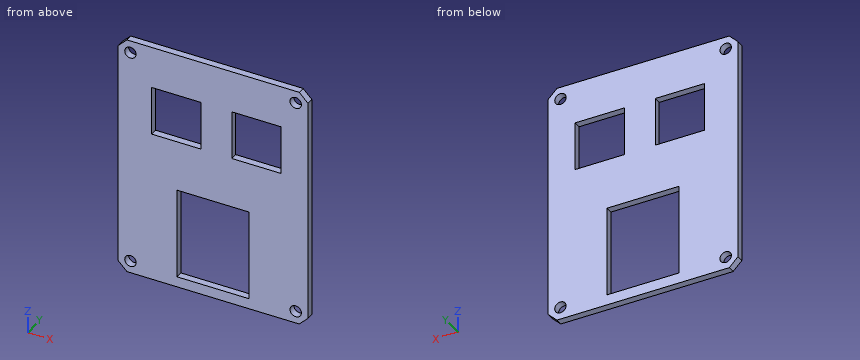
Autodesk Fusion 360 part; units mm, degrees
sketch "Sketch1" plane through (0, 0, 0) normal (0, 1, 0) x (1, 0, 0)
  line L0 (0, 0) -> (54, 0)
  line L1 (54, 0) -> (54, 69.5)
  line L2 (54, 69.5) -> (0, 69.5)
  line L3 (0, 69.5) -> (0, 0)
  dimension "d1" = 54
  dimension "d2" = 69.5
extrude "Extrude1" add sketch "Sketch1" along normal blind 2
chamfer "Chamfer1" distance 2.5 angle 45 4 edges at (54, 1, 0) (0, 1, 0) (54, 1, -69.5) (0, 1, -69.5)
sketch "Sketch2" plane through (0, 2, 0) normal (0, 1, 0) x (-1, 0, 0)
  line L0 (-2.5, -69.5) -> (0, -67)
  line L1 (0, -67) -> (0, -2.5)
  line L2 (0, -2.5) -> (-2.5, 0)
  line L3 (-2.5, 0) -> (-51.5, 0)
  line L4 (-51.5, 0) -> (-54, -2.5)
  line L5 (-54, -2.5) -> (-54, -67)
  line L6 (-54, -67) -> (-51.5, -69.5)
  line L7 (-51.5, -69.5) -> (-2.5, -69.5)
  line L8 (0, 0) -> (-3.5, 0)
  line L9 (-3.5, 0) -> (-3.5, -3.5)
  circle A0 centre (-3.5, -3.5) radius 1.625
  line L10 (-27, 0) -> (-27, -69.5)
  line L11 (0, -34.75) -> (-54, -34.75)
  circle A1 centre (-50.5, -3.5) radius 1.625
  circle A2 centre (-3.5, -66) radius 1.625
  circle A3 centre (-50.5, -66) radius 1.625
  dimension "d6" = 3.5
  dimension "d7" = 3.5
  dimension "d8" = 3.25
extrude "Extrude2" cut sketch "Sketch2" against normal blind 5 contours A0 | A1 | A2 | A3
sketch "Sketch3" plane through (0, 2, 0) normal (0, 1, 0) x (-1, 0, 0)
  circle A0 centre (-50.5, -3.5) radius 1.625
  circle A1 centre (-50.5, -66) radius 1.625
  circle A2 centre (-3.5, -3.5) radius 1.625
  circle A3 centre (-3.5, -66) radius 1.625
  line L0 (-2.5, -69.5) -> (0, -67)
  line L1 (0, -67) -> (0, -2.5)
  line L2 (0, -2.5) -> (-2.5, 0)
  line L3 (-2.5, 0) -> (-51.5, 0)
  line L4 (-51.5, 0) -> (-54, -2.5)
  line L5 (-54, -2.5) -> (-54, -67)
  line L6 (-54, -67) -> (-51.5, -69.5)
  line L7 (-51.5, -69.5) -> (-2.5, -69.5)
  line L8 (0, 0) -> (-16.5, 0)
  line L9 (-16.5, 0) -> (-16.5, -19)
  line L10 (-16.5, -19) -> (-39.35, -19)
  line L11 (-9.5, -12) -> (-23.5, -12)
  line L12 (-23.5, -12) -> (-23.5, -26)
  line L13 (-23.5, -26) -> (-9.5, -26)
  line L14 (-9.5, -26) -> (-9.5, -12)
  line L15 (-9.5, -12) -> (-23.5, -26) construction
  line L16 (-23.5, -12) -> (-9.5, -26) construction
  line L17 (-32.35, -26) -> (-46.35, -26)
  line L18 (-46.35, -26) -> (-46.35, -12)
  line L19 (-46.35, -12) -> (-32.35, -12)
  line L20 (-32.35, -12) -> (-32.35, -26)
  line L21 (-32.35, -26) -> (-46.35, -12) construction
  line L22 (-46.35, -26) -> (-32.35, -12) construction
  line L23 (0, 0) -> (-28.25, 0)
  line L24 (-28.25, 0) -> (-28.25, -40.5)
  line L25 (-28.25, -40.5) -> (-28.25, -66.5)
  line L26 (0, 0) -> (-18.25, 0)
  line L27 (-18.25, 0) -> (-18.25, -52)
  line L28 (-18.25, -52) -> (-16.75, -52)
  line L29 (-16.75, -52) -> (-28.25, -52)
  line L30 (-28.25, -52) -> (-28.25, -66.5)
  line L31 (-28.25, -66.5) -> (-16.75, -66.5)
  line L32 (-16.75, -66.5) -> (-16.75, -52)
  line L33 (-16.75, -52) -> (-28.25, -52)
  line L34 (-28.25, -52) -> (-28.25, -40.5)
  line L35 (-28.25, -40.5) -> (-16.75, -40.5)
  line L36 (-16.75, -40.5) -> (-16.75, -52)
  line L37 (0, 0) -> (-35.75, 0)
  line L38 (-35.75, 0) -> (-35.75, -44.5)
  line L39 (-35.75, -44.5) -> (-37.25, -44.5)
  line L40 (-37.25, -44.5) -> (-28.25, -44.5)
  line L41 (-28.25, -44.5) -> (-28.25, -40.5)
  line L42 (-28.25, -40.5) -> (-37.25, -40.5)
  line L43 (-37.25, -40.5) -> (-37.25, -44.5)
  line L44 (-37.25, -44.5) -> (-28.25, -44.5)
  line L45 (-28.25, -44.5) -> (-28.25, -66.5)
  line L46 (-28.25, -66.5) -> (-37.25, -66.5)
  line L47 (-37.25, -66.5) -> (-37.25, -44.5)
  point P0 (-16.5, -19)
  point P1 (-39.35, -19)
  dimension "d11" = 16.5
  dimension "d12" = 19
  dimension "d13" = 22.85
  dimension "d14" = 14
  dimension "d15" = 14
  dimension "d16" = 14
  dimension "d17" = 14
  dimension "d18" = 28.25
  dimension "d19" = 40.5
  dimension "d20" = 26
  dimension "d21" = 18.25
  dimension "d22" = 52
  dimension "d23" = 1.5
  dimension "d24" = 35.75
  dimension "d25" = 44.5
  dimension "d26" = 1.5
extrude "Extrude3" cut sketch "Sketch3" against normal blind 2 contours L9 L10 L11 L13 L14 L27 | L9 L10 L11 L27 | L10 L11 L12 L27 | L17 L18 L19 L38 | L10 L19 L20 L38 | L10 L12 L13 L27 | L10 L17 L20 L38 | L25 L27 L29 L33 L34 L35 L41 L45 | L25 L34 L38 L40 L41 L42 L44 | L25 L30 L34 L39 L40 L44 L45 L46 L47 | L27 L28 L29 L33 L35 L36 | L38 L39 L40 L42 L43 L44 | L25 L28 L29 L30 L31 L32 L33 L45
equation "d13 = 39.35 mm - 16.5 mm"
equation "d19 = 42 mm - 1.5 mm"
Verification items for the finished model (mm, model axes). Give positions to 0.01 mm unless a question says otherwise; leave off trailing zeros. Loops run counter-clockwise (first coordinate to the right, second up) from the corner with the lowest first, then second, coordinate; pieces in that order, holes last. Notation, with made-up numbers: (35, -34) - (62, -34) arc R16 cw to (62, -15) - close; hole circle Ø9 at (83.5, 10.5). An arc over 180 degrees is marked (long way). Write each question's results on one line, items separated by ' | '.
1) Depth check by flat-ended pin: P1, Ø3, axis at x = 50.5, z = -3.5, coming from the -Y side; P2, Ø1, axis at y = 0.5, z = -22, coming from the -X side. Enter the tip coordinate at first touch or a pass-through.
Solution:
P1: through | P2: x = 0
2) Sectioned sample at A-A on x = 26. Record the boundary of the cut face in (y, z), plus the area to 3 significant figures.
Solution:
outline: (0, -69.5) - (2, -69.5) - (2, -66.5) - (0, -66.5) - close; (0, -40.5) - (2, -40.5) - (2, 0) - (0, 0) - close | area: 87.0 mm2
3) Sectioned sample at C-C on y = 1.3. Record the boundary of the cut face in (x, z) (3 decimals).
Solution:
outline: (0, -67) - (2.5, -69.5) - (51.5, -69.5) - (54, -67) - (54, -2.5) - (51.5, 0) - (2.5, 0) - (0, -2.5) - close; hole circle Ø3.25 at (3.5, -66); hole circle Ø3.25 at (3.5, -3.5); hole (9.5, -26) - (23.5, -26) - (23.5, -12) - (9.5, -12) - close; hole (16.75, -66.5) - (37.25, -66.5) - (37.25, -40.5) - (16.75, -40.5) - close; hole (32.35, -26) - (46.35, -26) - (46.35, -12) - (32.35, -12) - close; hole circle Ø3.25 at (50.5, -66); hole circle Ø3.25 at (50.5, -3.5)
4) Material ranges on L1, parallel to X at y = 1, z = -66 (3 decimals); L2, parallel to Z at x = 34, y = 1.8; L3, parallel to Z at x = 50.5, y = 1.6 (3 decimals), recorded low to high. Write a range as from..to.
Solution:
L1: 0..1.875, 5.125..16.75, 37.25..48.875, 52.125..54 | L2: -69.5..-66.5, -40.5..-26, -12..0 | L3: -69.5..-67.625, -64.375..-5.125, -1.875..0
5) Sectioned sample at B-B on z = -24.5. Record the boundary of the cut face in (x, y).
Solution:
outline: (0, 0) - (9.5, 0) - (9.5, 2) - (0, 2) - close; (23.5, 0) - (32.35, 0) - (32.35, 2) - (23.5, 2) - close; (46.35, 0) - (54, 0) - (54, 2) - (46.35, 2) - close
6) Sectioned sample at D-D on x = 50.5. Record the boundary of the cut face in (y, z) (3 decimals).
Solution:
outline: (0, -69.5) - (2, -69.5) - (2, -67.625) - (0, -67.625) - close; (0, -64.375) - (2, -64.375) - (2, -5.125) - (0, -5.125) - close; (0, -1.875) - (2, -1.875) - (2, 0) - (0, 0) - close
